Here's how the part is built. I have some questions about the finished solid (model axes, mm). A direction names the side the tool comes from. Coordinates: 2 decimals unless noted, no trailing zeros. Loops run counter-clockwise (first coordinate to the right, second up) from the corner with the lowest first, then second, coordinate; pieces in that order, holes last. Notation, with made-up numbers: (18, -7) -> (61, -7) arc R16 cw to (61, 2) -> close; hole circle Ø6 at (-9, 64.5). An arc over 180 degrees is marked (long way). Answer as a JSON object with one key per item and string values. Group by question number.
1) I want a section at A-A (y = 0). Write out the boundary of the cut face in (x, z), then the cut area to 3 significant figures.
2) I'm going to push flat-ended pins straight in: pin 1 (1 mm diameter, centred on y = 7.5, z = 18.5, fed in from -X) (3 decimals); pin 2 (2 mm diameter, centred on y = -5.5, z = 79.5, fed in from -X); pin 3 (4 mm diameter, centred on x = 17, z = 5.5, fed in from +Y). Where does each tip first touch, or does it pass through?
3) Which directions (+Z, -Z, +X, -X, +Y, -Y) give clear straight access to the entire face, cutting with the end or side of a thin tool? Please do faces 5 (the flat face through (-6.8, 10.7, 100)), 6 (the cylindrical face through (-12.488, 0.55, 49.3)).
4) I want a section at C-C (x = 0). Write out the boundary of the cut face in (y, z).
5) I need wall thicknesses on probe 1 along X at (y, z) = (0, 51); probe 2 along Z at (x, y) = (-43, -16); probe 3 along Z at (x, y) = (-16, 0). Which ranges of each line are inside material? Lowest first, please. Write a range as [from, to].
6) I want a section at B-B (z = 37.5). Write out the boundary of the cut face in (x, y).
7) If we mould it in two halves opening along Z, with no side actions, what happens to faces 1 (the cylindrical face through (-14.93, 6.93, 34.63)), 2 (the flat face through (0, 0, 0)), 3 (the flat face through (50, 0, -5)), 4 (the flat face through (-1, 0, -10))? For each: +Z half, -Z half, draft (parallel to the pull), parting line (faces both ways), or undercut.
8) I want a section at D-D (z = 88.5). Write out the boundary of the cut face in (x, y).
```python
from build123d import *

# Parameters (mm, degrees)
F0_R     = 20
F0_R_2   = 12.5
F1_DEPTH = 100
F2_W     = 100
F2_H     = 60
F3_DEPTH = 10
F4_R     = 5
F5_SIZE  = 7
F6_R     = 7.5
F7_DEPTH = 20


with BuildPart() as f1:
    # F0 (on Top) → F1 (new body)
    with BuildSketch(Plane.XY):
        Circle(F0_R)
        Circle(F0_R_2, mode=Mode.SUBTRACT)
    extrude(amount=F1_DEPTH)

    # F2 (on Top) → F3 (join)
    with BuildSketch(Plane.XY):
        Rectangle(F2_W, F2_H)
    extrude(amount=-F3_DEPTH)

    # F4
    f4_edges = [f1.edges().sort_by_distance(p)[0] for p in [
        (-50, -30, -5),
        (50, -30, -5),
        (50, 30, -5),
        (-50, 30, -5),
    ]]
    fillet(f4_edges, radius=F4_R)

    # F5
    f5_edges = [f1.edges().sort_by_distance(p)[0] for p in [
        (-20, 0, 100),
    ]]
    chamfer(f5_edges, length=F5_SIZE)

    # F6 (on Right) → F7 (cut, symmetric)
    with BuildSketch(Plane.YZ):
        with Locations((0, 37.5)):
            Circle(F6_R)
    extrude(amount=F7_DEPTH, both=True, mode=Mode.SUBTRACT)


solid = f1.part
```
Determined:
{
 "1": {"outline": "(-50, -10) -> (50, -10) -> (50, 0) -> (20, 0) -> (20, 30) -> (12.5, 30) -> (12.5, 0) -> (-12.5, 0) -> (-12.5, 30) -> (-20, 30) -> (-20, 0) -> (-50, 0) -> close; (-20, 45) -> (-12.5, 45) -> (-12.5, 100) -> (-13, 100) -> (-20, 93) -> close; (12.5, 45) -> (20, 45) -> (20, 93) -> (13, 100) -> (12.5, 100) -> close", "area": "2,230 mm^2"},
 "2": {"pin 1": "x = -18.735", "pin 2": "x = -19.49", "pin 3": "y = 13.23"},
 "3": {"face 5": "+Z, +X, -X, +Y, -Y", "face 6": "+Z"},
 "4": {"outline": "(-30, -10) -> (30, -10) -> (30, 0) -> (20, 0) -> (20, 93) -> (13, 100) -> (12.5, 100) -> (12.5, 0) -> (-12.5, 0) -> (-12.5, 100) -> (-13, 100) -> (-20, 93) -> (-20, 0) -> (-30, 0) -> close"},
 "5": {"probe 1": "[-20, -12.5], [12.5, 20]", "probe 2": "[-10, 0]", "probe 3": "[-10, 30], [45, 97]"},
 "6": {"outline": "(-18.54, -7.5) arc R20 ccw to (18.54, -7.5) -> (10, -7.5) arc R12.5 cw to (-10, -7.5) -> close; (-18.54, 7.5) -> (-10, 7.5) arc R12.5 cw to (10, 7.5) -> (18.54, 7.5) arc R20 ccw to start"},
 "7": {"face 1": "undercut", "face 2": "+Z half", "face 3": "draft", "face 4": "-Z half"},
 "8": {"outline": "circle Ø40 at (0, 0); hole circle Ø25 at (0, 0)"}
}
